Drawing for the job (mm, zero at the part's lowest x, y, z). A direction names the side the tool comes from. Round coordinates to 2 decimals unless told otherwise and drop trailing zeros. Write each loop counter-clockwise with the first axis right and the second up, starting at its lowest first coordinate (ties: lowest second). Pieces come first, ordered by that corner, then holes. Notation, with made-up numbers: M 59,0.25 L 86,0.25 A18 cw 86,26.25 Z; hole C -33.75,68.5 d2. An arc over 180 degrees is marked long. Use a Markdown table: item, result. Add a question column.
1) Two-plate mould, pull along Y, no slides. Class the marked faces 4, 5 and 6: released by +Y, released by -Y, zero draft, split by the parting line, or undercut.
2) Slice it at A-A on x = 9.75. Write the cut outline in (y, z).
3) Wall check: probe 1 along Z at (x, y) = (10.5, 6.55); probe 2 along X at (y, z) = (10, 3); probe 3 along Y at (x, z) = (0.5, 8) (1 decimal). Give the ranges that are in metal, low to high.
4) Slice it at B-B on x = 4.25. Write the cut outline in (y, z), plus the area to 3 significant figures.
5) Which spindle directions (+Z, -Z, +X, -X, +Y, -Y) get a long thin tool onto all of the face, cutting with end or side? Do the marked faces 1, 2 and 3. Say none if no direction does.
6) Drop flat-ended pins along their axis: P1, Ø5, axis at x = 9, y = 3.5, coming from the +Z side; P2, Ø1.1, axis at x = 0.5, z = 7, coming from the -Y side; P3, Ø1.5, axis at x = 7, y = 2.5, coming from the +Z side. Give the stop position or say it passes through.
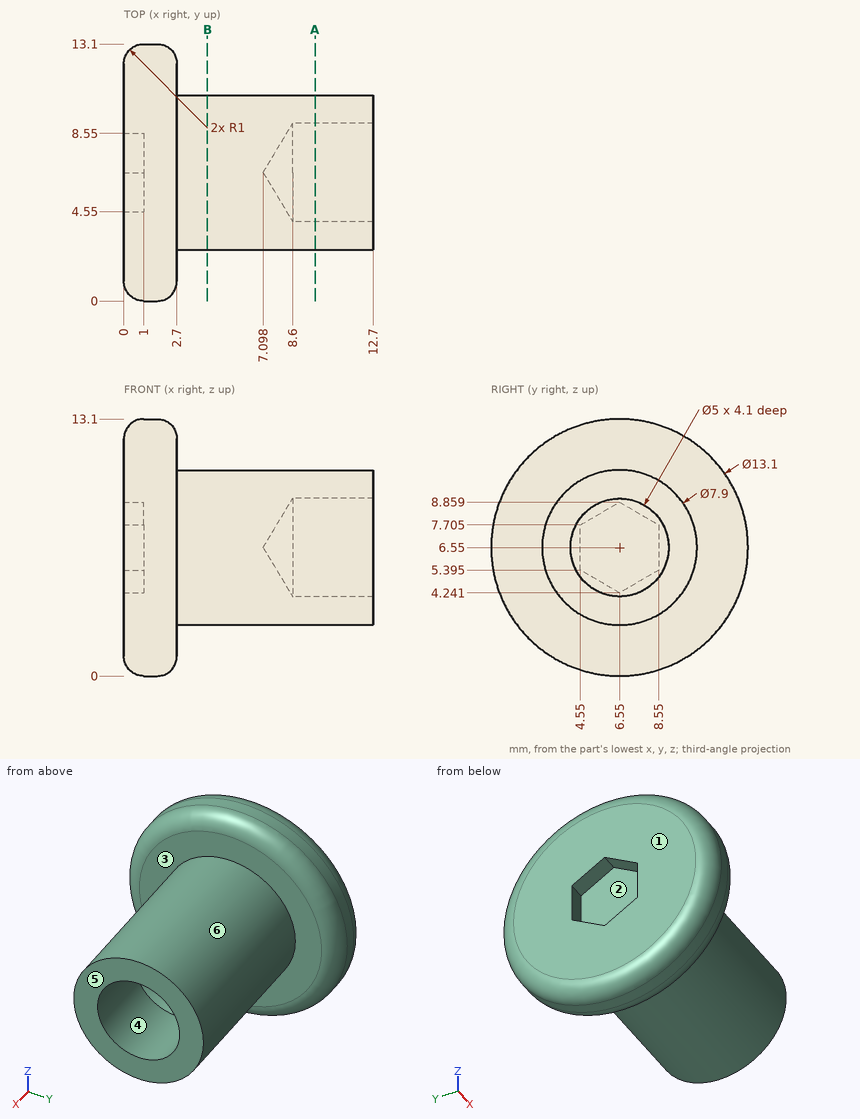
Entries:
| question | item | result |
|---|---|---|
| 1 | face 4 | undercut |
| 1 | face 5 | zero draft |
| 1 | face 6 | split by the parting line |
| 2 | outline | C 6.55,6.55 d7.9; hole C 6.55,6.55 d5 |
| 3 | probe 1 | z = 2.6 to 4.05, 9.05 to 10.5 |
| 3 | probe 2 | x = 0 to 2.7 |
| 3 | probe 3 | y = 0.3 to 5.1, 8 to 12.8 |
| 4 | outline | C 6.55,6.55 d7.9 |
| 4 | area | 49.0 mm^2 |
| 5 | face 1 | +Z, -Z, -X, +Y, -Y |
| 5 | face 2 | -X |
| 5 | face 3 | +X |
| 6 | P1 | stops at z = 10.46 |
| 6 | P2 | stops at y = 0 |
| 6 | P3 | stops at z = 8.72 |
